The listing builds one solid part. Answer for the finished solid, in the listing's coordinates (mm). A direction names the side the tool comes from. Give positions to 0.01 mm unless a question says otherwise; leave off trailing zeros. Loops run counter-clockwise (first coordinate to the right, second up) from the corner with the lowest first, then second, coordinate; pieces in that order, holes last.
Item 1: This flat-tipped pin is pushed along its axis until it touches: pin 1 Ø6 at (x, z) = (-14.5, 15) entering from +Y. Where does it stop, or does it pass through?
Item 2: Section A-A, the plane z = 23.5 is taken. Give the vertices of the cut face in (x, y).
Item 3: Section D-D, the plane z = 34.5 is taken. Give the vertices of the cut face in (x, y).
Item 4: The mould has two halves that part along Z. Classify faces 4 (the face through (20, 122, 20)), 5 (the face through (15.15, 123, 20)), 6 (the face through (0, 123, 0)): pulls with the +Z half, pulls with the -Z half, needs draft (parallel to the pull), parting line crosses it, or undercut.
Item 5: Section C-C, the plane x = -8 is taken. Give the vertices of the cut face in (y, z).
Item 6: Section B-B, the plane y = 122.8 is taken. Give the vertices of the cut face in (x, z), and give its area (3 significant figures).
Item 7: Consider line 1 along X through (y, z) = (120.55, 25); line 2 along Z through (x, y) = (5.5, 120.85); line 3 along Z through (x, y) = (5.5, 123.45). Determine where each line is inside the solid, lowest interval first.
Item 8: A tool of negligible diameter and unlimited length cuts with its end or side. For faces 1 (the face through (-15.15, 123, 20)), 2 (the face through (0, 121, 10)), 3 (the face through (0, 125, 37)), from which of +Z, -Z, +X, -X, +Y, -Y can it reach the whole face along a straight path? Write none if from no direction.
Autodesk Inventor part; units mm, degrees
ref_plane "YZ Plane" through (0, 0, 0) normal (1, 0, 0) x (0, 1, 0)
ref_plane "XZ Plane" through (0, 0, 0) normal (0, 1, 0) x (-1, 0, 0)
ref_plane "XY Plane" through (0, 0, 0) normal (0, 0, 1) x (1, 0, 0)
sketch "Sketch1" plane through (0, 0, 0) normal (0, 0, 1) x (1, 0, 0)
  arc A0 (20, 123.3896) -> (-20, 123.3896) centre (0, 0) ccw
  line L0 (20, 120) -> (-20, 120)
  line L1 (-20, 120) -> (-20, 123.3896)
  line L2 (20, 120) -> (20, 123.3896)
  line L3 (0, 0) -> (0, 32.1156) construction
  point P0 (0, 125)
  dimension "d0" = 250
  dimension "d1" = 40
  dimension "d2" = 5
extrude "Extrusion1" add sketch "Sketch1" along normal blind 40
sketch "Sketch2" plane through (-20, 120, 0) normal (0, -1, 0) x (1, 0, 0)
  line L0 (4.85, 4.85) -> (35.15, 4.85)
  line L1 (35.15, 4.85) -> (35.15, 35.15)
  line L2 (35.15, 35.15) -> (4.85, 35.15)
  line L3 (4.85, 35.15) -> (4.85, 4.85)
  line L4 (4.85, 4.85) -> (35.15, 35.15) construction
  line L5 (35.15, 4.85) -> (4.85, 35.15) construction
  line L6 (40, 0) -> (40, 40)
  line L7 (40, 0) -> (0, 0)
  point P0 (20, 0)
  point P1 (20, 20)
  point P2 (40, 20)
  point P3 (20, 0)
  dimension "d6" = 30.3
  dimension "d7" = 30.3
extrude "Extrusion2" cut sketch "Sketch2" against normal blind 30
sketch "Sketch3" plane through (-20, 120, 0) normal (0, -1, 0) x (1, 0, 0)
  line L0 (35.15, 35.15) -> (35.15, 4.85)
  line L1 (4.85, 35.15) -> (35.15, 35.15)
  line L2 (35.15, 35.15) -> (35.15, 4.85)
  line L3 (35.15, 4.85) -> (4.85, 4.85)
  line L4 (4.85, 4.85) -> (4.85, 35.15)
  line L5 (4.85, 35.15) -> (35.15, 4.85) construction
  line L6 (35.15, 35.15) -> (4.85, 4.85) construction
  line L7 (10, 10) -> (30, 10)
  line L8 (30, 10) -> (30, 30)
  line L9 (30, 30) -> (10, 30)
  line L10 (10, 30) -> (10, 10)
  line L11 (10, 10) -> (30, 30) construction
  line L12 (30, 10) -> (10, 30) construction
  point P0 (20, 0)
  point P1 (20, 20)
  dimension "d10" = 20
extrude "Extrusion3" add sketch "Sketch3" against normal blind 2
properties part number "cooler_plate_socket" material "Acetal Resin, Black"
Worked answers:
1. pin 1: stops at y = 124.08
2. outline: (-20, 120) - (-10, 120) - (-10, 122) - (-15.15, 122) - (-15.15, 124.08) arc R125 ccw to (-20, 123.39) - close; (10, 120) - (20, 120) - (20, 123.39) arc R125 ccw to (15.15, 124.08) - (15.15, 122) - (10, 122) - close
3. outline: (-20, 120) - (20, 120) - (20, 123.39) arc R125 ccw to (15.15, 124.08) - (15.15, 122) - (-15.15, 122) - (-15.15, 124.08) arc R125 ccw to (-20, 123.39) - close
4. face 4: needs draft
4. face 5: undercut
4. face 6: pulls with the -Z half
5. outline: (120, 0) - (124.74, 0) - (124.74, 4.85) - (122, 4.85) - (122, 10) - (120, 10) - close; (120, 30) - (122, 30) - (122, 35.15) - (124.74, 35.15) - (124.74, 40) - (120, 40) - close
6. outline: (-20, 0) - (20, 0) - (20, 40) - (-20, 40) - close; hole (-15.15, 4.85) - (15.15, 4.85) - (15.15, 35.15) - (-15.15, 35.15) - close
6. area: 682 mm2
7. line 1: x = -20 to -10, 10 to 20
7. line 2: z = 0 to 10, 30 to 40
7. line 3: z = 0 to 4.85, 35.15 to 40
8. face 1: +Y
8. face 2: +Y, -Y
8. face 3: +Z, -Z, +Y
